from build123d import *

# Parameters (mm, degrees)
F0_W     = 7.2
F0_H     = 4
F0_W_2   = 40.6
F0_H_2   = 6
F0_H_3   = 28
F1_DEPTH = 10
F3_D     = 4
F4_SIZE  = 5


# Not quite as in the source:
# - the program builds the solid bodies; features that only make, move or delete a surface that nothing else refers to are left out


with BuildPart() as f1:
    # F0 (on Right) → F1 (new body, symmetric)
    with BuildSketch(Plane.YZ):
        with Locations((23.9, 9.8437508568)):
            Rectangle(F0_W, F0_H)
        with Locations((0, 14.8437508568)):
            Rectangle(F0_W_2, F0_H_2)
        with Locations((0, -6.1562491432)):
            Rectangle(F0_W_2, F0_H_3)
        with Locations((-23.9, 9.8437508568)):
            Rectangle(F0_W, F0_H)
        with Locations((0, 9.8437508568)):
            Rectangle(F0_W_2, F0_H)
    extrude(amount=F1_DEPTH, both=True)

    # F3 (through all)
    with Locations(Plane(origin=(0, 0, 0), x_dir=(1, 0, 0), z_dir=(0, 0, -1))):
        with Locations((-5, -25), (5, -25), (5, 25), (-5, 25)):
            Hole(F3_D / 2)

    # F4
    f4_edges = [f1.edges().sort_by_distance(p)[0] for p in [
        (0, -20.3, 17.843751),
        (0, 20.3, 17.843751),
    ]]
    chamfer(f4_edges, length=F4_SIZE)


solid = f1.part
Can you work these out from the model? Positions are in its coordinate system, mm. A direction names the side the tool comes from. Coordinates: 2 decimals unless noted, no trailing zeros. Write each loop counter-clockwise with the first axis right and the second up, starting at its lowest first coordinate (ties: lowest second). Pieces come first, ordered by that corner, then holes. Notation, with made-up numbers: (76.5, 60.25) -> (102.5, 60.25) arc R20 cw to (102.5, 84.25) -> close; hole circle Ø6 at (48.5, 73). An arc over 180 degrees is marked (long way). Answer as CSV lines item,"result".
1) If we section it at D-D on x = 9: Please give me the cut outline in (y, z), then the cut area to 3 significant figures.
Check result:
outline,"(-27.5, 7.84) -> (-20.3, 7.84) -> (-20.3, -20.16) -> (20.3, -20.16) -> (20.3, 7.84) -> (27.5, 7.84) -> (27.5, 11.84) -> (20.3, 11.84) -> (20.3, 12.84) -> (15.3, 17.84) -> (-15.3, 17.84) -> (-20.3, 12.84) -> (-20.3, 11.84) -> (-27.5, 11.84) -> close"
area,"1,580 mm²"
2) If we section it at A-A on x = -5: Please give me the cut outline in (y, z), then the cut area to 3 significant figures.
Check result:
outline,"(-27.5, 7.84) -> (-27, 7.84) -> (-27, 11.84) -> (-27.5, 11.84) -> close; (-23, 7.84) -> (-20.3, 7.84) -> (-20.3, -20.16) -> (20.3, -20.16) -> (20.3, 7.84) -> (23, 7.84) -> (23, 11.84) -> (20.3, 11.84) -> (20.3, 12.84) -> (15.3, 17.84) -> (-15.3, 17.84) -> (-20.3, 12.84) -> (-20.3, 11.84) -> (-23, 11.84) -> close; (27, 7.84) -> (27.5, 7.84) -> (27.5, 11.84) -> (27, 11.84) -> close"
area,"1,540 mm²"
3) On a 3-axis mill with a long thin cutter (end or side, diameter ignored), from which of +Z, -Z, +X, -X, +Y, -Y can I reach the whole of each face in a straight line? I mean faces 1 (the cylindrical face through (-3.4, 26.2, 9.9)), 2 (the flat face through (0, 24, 7.844)), 3 (the flat face through (-0.14, 17.765, 15.379)), 4 (the flat face through (0, -24, 11.844)), 5 (the flat face through (0, -24, 7.844)). Say none if no direction works.
Check result:
face 1,"+Z, -Z"
face 2,"-Z, +X, -X, +Y"
face 3,"+Z, +X, -X, +Y"
face 4,"+Z, +X, -X, -Y"
face 5,"-Z, +X, -X, -Y"
4) If I drill on line 1 (Y direction, x = -5, z = 10.85); line 2 (X direction, y = -25, z = 8); line 3 (Y direction, x = 2.5, z = -7.5), over which ranges is the centre line in solid material (lowest first)? Write a range as from..to.
Check result:
line 1,"-27.5..-27, -23..23, 27..27.5"
line 2,"-10..-7, -3..3, 7..10"
line 3,"-20.3..20.3"
5) If we section it at C-C on z = 9.5: Please give me the cut outline in (x, y), then the cut area to 3 significant figures.
Check result:
outline,"(-10, -27.5) -> (10, -27.5) -> (10, 27.5) -> (-10, 27.5) -> close; hole circle Ø4 at (-5, -25); hole circle Ø4 at (-5, 25); hole circle Ø4 at (5, -25); hole circle Ø4 at (5, 25)"
area,"1,050 mm²"
6) Will these pins go through, and if not, where does the flat tip stop? P1, Ø1, axis at x = 0.5, y = 21, coming from the -Z side; P2, Ø1, axis at x = 1, z = -7.5, coming from the -Y side; P3, Ø0.8, axis at x = -2, z = 12.5, coming from the +Y side.
Check result:
P1,"z = 7.84"
P2,"y = -20.3"
P3,"y = 20.3"
7) If we section it at B-B on y = -25: Please give me the cut outline in (x, z).
Check result:
outline,"(-10, 7.84) -> (-7, 7.84) -> (-7, 11.84) -> (-10, 11.84) -> close; (-3, 7.84) -> (3, 7.84) -> (3, 11.84) -> (-3, 11.84) -> close; (7, 7.84) -> (10, 7.84) -> (10, 11.84) -> (7, 11.84) -> close"
8) If we mould it in two halves opening along X, with no side actions, what happens to faces 6 (the flat face through (0, 24, 11.844)), 7 (the flat face through (-10, 0, -1)), 8 (the cylindrical face through (5, -23, 10))? For each: +X half, -X half, draft (parallel to the pull), parting line (faces both ways), or undercut.
Check result:
face 6,"draft"
face 7,"-X half"
face 8,"undercut"
